from build123d import *

# Parameters (mm, degrees)
SKETCH1_R               = 1.778
BOSS_EXTRUDE1_DEPTH     = 6.35
CUT_EXTRUDE1_DEPTH      = 45.59065674
CUT_EXTRUDE1_DEPTH_BACK = 45.59065674
SKETCH2_W               = 15.126003495
SKETCH2_H               = 9.710924743
FILLET1_R               = 4.7625


with BuildPart() as part:
    # Sketch1 → Boss-Extrude1 (new body)
    with BuildSketch(Plane.XZ):
        with BuildLine():
            Line((-39.116, -4.7625), (39.116, -4.7625))
            ThreePointArc((39.116, -4.7625), (43.8785, 0), (39.116, 4.7625))
            Line((39.116, 4.7625), (-39.116, 4.7625))
            ThreePointArc((-39.116, 4.7625), (-43.8785, 0), (-39.116, -4.7625))
        make_face()
        with Locations(Location((39.116, 0, 0), (0, 0, 90))):
            Circle(SKETCH1_R, mode=Mode.SUBTRACT)
        with Locations(Location((29.337, 0, 0), (0, 0, 90))):
            Circle(SKETCH1_R, mode=Mode.SUBTRACT)
        with Locations(Location((19.558, 0, 0), (0, 0, 90))):
            Circle(SKETCH1_R, mode=Mode.SUBTRACT)
        with Locations(Location((9.779, 0, 0), (0, 0, 90))):
            Circle(SKETCH1_R, mode=Mode.SUBTRACT)
        with Locations(Location((0, 0, 0), (0, 0, 90))):
            Circle(SKETCH1_R, mode=Mode.SUBTRACT)
        with Locations(Location((-9.779, 0, 0), (0, 0, 90))):
            Circle(SKETCH1_R, mode=Mode.SUBTRACT)
        with Locations(Location((-19.558, 0, 0), (0, 0, 90))):
            Circle(SKETCH1_R, mode=Mode.SUBTRACT)
        with Locations(Location((-29.337, 0, 0), (0, 0, 90))):
            Circle(SKETCH1_R, mode=Mode.SUBTRACT)
        with Locations(Location((-39.116, 0, 0), (0, 0, 90))):
            Circle(SKETCH1_R, mode=Mode.SUBTRACT)
    extrude(amount=-BOSS_EXTRUDE1_DEPTH)

    # Sketch2 → Cut-Extrude1 (cut, two sides: drawn at the far end of the back side and taken through both)
    with BuildSketch(Plane(origin=(0, 6.35, 0), x_dir=(1, 0, 0), z_dir=(0, 1, 0)).offset(-CUT_EXTRUDE1_DEPTH_BACK)):
        with Locations((-41.662501748, 0.092962372)):
            Rectangle(SKETCH2_W, SKETCH2_H)
    extrude(amount=CUT_EXTRUDE1_DEPTH + CUT_EXTRUDE1_DEPTH_BACK, mode=Mode.SUBTRACT)

    # Fillet1
    fillet1_edges = [part.edges().sort_by_distance(p)[0] for p in [
        (-34.0995, 3.175, -4.7625),
        (-34.0995, 3.175, 4.7625),
    ]]
    fillet(fillet1_edges, radius=FILLET1_R - 0.0001)  # a hair under: the kernel refuses the full size


solid = part.part
Model file for the job. Use its own axes, mm. Give positions to 0.01 mm unless a question says otherwise; leave off trailing zeros. Loops run counter-clockwise (first coordinate to the right, second up) from the corner with the lowest first, then second, coordinate; pieces in that order, holes last. Notation, with made-up numbers: (-1, 54.25) -> (10, 54.25) arc R22 ccw to (10, 87.25) -> close; hole circle Ø10 at (65, 65.25). An arc over 180 degrees is marked (long way). Use a Markdown table: item, result. Add a question column.
(1) Slice it at D-D on z = -2.5. List the corners of the cut face in (x, y).
(2) Mould opens along Z. For faces 1 (the cylindrical face through (21.294, 3.131, -0.385)), 2 (the flat face through (4, 0, 0)), 3 (the cylindrical face through (1.736, 3.131, -0.385)), 4 (the flat face through (5, 3, 4.762)) say: +Z half, -Z half, draft (parallel to the pull), parting line (faces both ways), or undercut.
(3) Slice it at A-A on x = 0. List the corners of the cut face in (y, z).
(4) Slice it at B-B on y = 3.25. Give the number of separate pieces and of enclosed holes in the cut face, and give its area (3 significant figures).
(5) Wall check: line 1 along Z through (x, y) = (10, 1.5); line 2 along Z through (x, y) = (30, 1); line 3 along X through (y, z) = (3.25, -4). Give the ranges that are in metal, low to high.
(6) Drop flat-ended pins along their axis: pin 1 Ø3 at (x, z) = (0, 0) entering from -Y; pin 2 Ø3 at (y, z) = (4, -3.5) entering from -X; pin 3 Ø1 at (y, z) = (5.5, -3) entering from +X. Give the stop position or say it passes through.
Filled sheet:
| question | item | result |
|---|---|---|
| 1 | outline | (-33.39, 0) -> (43.17, 0) -> (43.17, 6.35) -> (-33.39, 6.35) -> close |
| 2 | face 1 | undercut |
| 2 | face 2 | draft |
| 2 | face 3 | undercut |
| 2 | face 4 | +Z half |
| 3 | outline | (0, -4.76) -> (6.35, -4.76) -> (6.35, -1.78) -> (0, -1.78) -> close; (0, 1.78) -> (6.35, 1.78) -> (6.35, 4.76) -> (0, 4.76) -> close |
| 4 | separate pieces | 1 |
| 4 | enclosed holes | 8 |
| 4 | area | 644 mm2 |
| 5 | line 1 | -4.76 to -1.76, 1.76 to 4.76 |
| 5 | line 2 | -4.76 to -1.65, 1.65 to 4.76 |
| 5 | line 3 | -31.92 to 41.7 |
| 6 | pin 1 | through |
| 6 | pin 2 | x = -33.66 |
| 6 | pin 3 | x = 43.17 |
